```python
from build123d import *

# Parameters (mm, degrees)
F0_R     = 63.5
F1_DEPTH = 76.2
F2_T     = -12.7
F3_R     = 6.34999


# Not quite as in the source:
# - a fillet or chamfer is up to 0.001 mm smaller than in the source, because OpenCascade refuses the exact size


with BuildPart() as f1:
    # F0 (on Front) → F1 (new body)
    with BuildSketch(Plane.XZ):
        Circle(F0_R)
    extrude(amount=F1_DEPTH)

    # F2
    f2_openings = [f1.faces().sort_by_distance(p)[0] for p in [
        (0, 0, 0),
    ]]
    offset(amount=F2_T, openings=f2_openings)

    # F3 (radius 6.35 in the source; OpenCascade refuses exactly that, so slightly less here)
    f3_edges = [f1.edges().sort_by_distance(p)[0] for p in [
        (-63.5, 0, 0),
        (-50.8, 0, 0),
    ]]
    fillet(f3_edges, radius=F3_R)


solid = f1.part
```
The listing builds one solid part. Answer for the finished solid, in the listing's coordinates (mm). Give positions to 0.01 mm unless a question says otherwise; leave off trailing zeros. Write each loop counter-clockwise with the first axis right and the second up, starting at its lowest first coordinate (ties: lowest second). Pieces come first, ordered by that corner, then holes. Notation, with made-up numbers: (-36.5, 21) - (-29.5, 21) arc R29 cw to (-29.5, 52) - close; hole circle Ø4 at (72, -33.5). An arc over 180 degrees is marked (long way). Use one line per item in the form item = value. Start each with the question number.
1) Find section C-C on y = -33. Determine the outline of the cut face in (x, z), plus the area to 3 significant figures.
2) The mould has two halves that part along Z. Classify faces 1 (the face through (-13.77, -40.79, -61.99)), 2 (the face through (-1, -63.5, 1)), 3 (the face through (-11.012, -34.525, -49.592)), 4 (the face through (-1, -76.2, 1)): pulls with the +Z half, pulls with the -Z half, needs draft (parallel to the pull), parting line crosses it, or undercut.
3) Find section D-D on y = -66.5. Determine the outline of the cut face in (x, z), plus the area to 3 significant figures.
4) Consider line 1 along Z through (x, y) = (0, -47); line 2 along Y through (x, z) = (19, 3); line 3 along Z through (x, y) = (-8.5, -13.5). Determine where each line is inside the solid, lowest interval first. Write a range as from..to.
5) Flat-ended cylindrical pins translate along their axes: pin 1 Ø12 at (x, y) = (-5, -54) entering from +Z; pin 2 Ø1 at (x, y) = (-31, -14.5) entering from -Z; pin 3 Ø5 at (x, y) = (-47.5, -15.5) entering from +Z. Find the tip coordinate at first contact, or state that the pin passes through.
Geometry results:
q1.outline = circle Ø127 at (0, 0); hole circle Ø101.6 at (0, 0)
q1.area = 4,560 mm2
q2.face_1 = parting line crosses it
q2.face_2 = undercut
q2.face_3 = undercut
q2.face_4 = needs draft
q3.outline = circle Ø127 at (0, 0)
q3.area = 12,700 mm2
q4.line_1 = -63.5..-50.8, 50.8..63.5
q4.line_2 = -76.2..-63.5
q4.line_3 = -62.93..-50.08, 50.08..62.93
q5.pin_1 = 63.5
q5.pin_2 = -55.7
q5.pin_3 = 44.8
